```python
from build123d import *

# Parameters (mm, degrees)
SKETCH1_W           = 100
SKETCH1_H           = 80
BOSS_EXTRUDE1_DEPTH = 55
SKETCH3_W           = 90
SKETCH3_H           = 70
CUT_EXTRUDE1_DEPTH  = 50
SKETCH5_R           = 1.5
CUT_EXTRUDE2_DEPTH  = 50


with BuildPart() as part:
    # Sketch1 → Boss-Extrude1 (new body)
    with BuildSketch(Plane(origin=(0, 0, 0), x_dir=(1, 0, 0), z_dir=(0, 1, 0))):
        Rectangle(SKETCH1_W, SKETCH1_H)
    extrude(amount=BOSS_EXTRUDE1_DEPTH)

    # Sketch3 → Cut-Extrude1 (cut)
    with BuildSketch(Plane(origin=(0, 55, 0), x_dir=(1, 0, 0), z_dir=(0, 1, 0))):
        Rectangle(SKETCH3_W, SKETCH3_H)
    extrude(amount=-CUT_EXTRUDE1_DEPTH, mode=Mode.SUBTRACT)

    # Sketch5 → Cut-Extrude2 (cut)
    with BuildSketch(Plane(origin=(0, 5, 0), x_dir=(1, 0, 0), z_dir=(0, 1, 0))):
        with Locations(Location((-34.701504138, 23.983302554, 0), (0, 0, 270))):
            Circle(SKETCH5_R)
        with Locations(Location((34.701504138, 23.983302554, 0), (0, 0, 270))):
            Circle(SKETCH5_R)
        with Locations(Location((34.701504138, -23.983302554, 0), (0, 0, 270))):
            Circle(SKETCH5_R)
        with Locations(Location((-34.701504138, -23.983302554, 0), (0, 0, 270))):
            Circle(SKETCH5_R)
    extrude(amount=-CUT_EXTRUDE2_DEPTH, mode=Mode.SUBTRACT)


solid = part.part
```
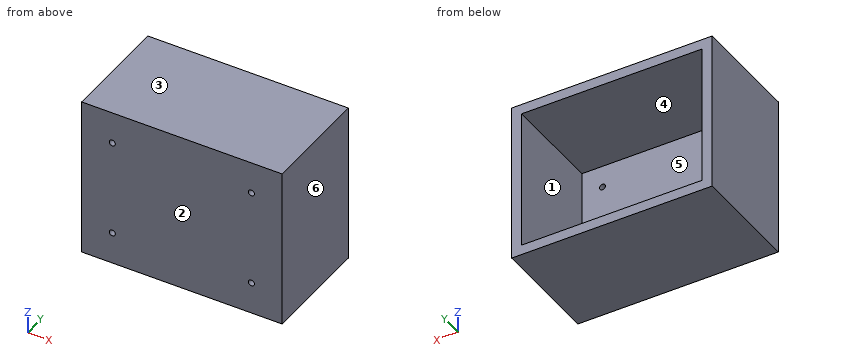
CAD build for the part. Positions are in the model's coordinates, mm. Face numbers are marked on the shaded views. A direction names the side the tool comes from. Coordinates: 2 decimals unless noted, no trailing zeros. Write each loop counter-clockwise with the first axis right and the second up, starting at its lowest first coordinate (ties: lowest second). Pieces come first, ordered by that corner, then holes. Notation, with made-up numbers: (-11.75, 80.5) -> (40.25, 80.5) arc R20 cw to (40.25, 94.5) -> close; hole circle Ø2 at (70.5, 33). An arc over 180 degrees is marked (long way). Use CSV: the item, a comma, the result in double quotes. Start each with the question number.
Item 1: Band-saw the part on A-A, the plane y = 32. Write the cut outline in (x, z), plus the area to 3 significant figures.
Item 2: Tool access for the marked faces 5 and 6: list every direction of +Z, -Z, +X, -X, +Y, -Y with a clear straight run to the whole face (end or side of a thin tool).
Item 3: Band-saw the part on C-C, the plane x = 22.5. Write the cut outline in (y, z), plus the area to 3 significant figures.
Item 4: Two-plate mould, pull along Z, no slides. Class the marked faces 1, 2, 3 and 4: +Z half, -Z half, draft (parallel to the pull), parting line (faces both ways), or undercut.
Item 5: Band-saw the part on B-B, the plane z = 4.5. Write the cut outline in (x, y), plus the area to 3 significant figures.
Item 6: Wall check: probe 1 along X at (y, z) = (48.5, 1); probe 2 along Z at (x, y) = (32, 27.5); probe 3 along X at (y, z) = (2.5, -24.5). Give the ranges that are in metal, low to high.
Item 7: Drop a flat-ended pin along its axis: P1, Ø1, axis at x = -28, z = -1, coming from the +Y side. Give the stop position or say it passes through.
Response values:
1,outline,"(-50, -40) -> (50, -40) -> (50, 40) -> (-50, 40) -> close; hole (-45, -35) -> (45, -35) -> (45, 35) -> (-45, 35) -> close"
1,area,"1,700 mm2"
2,face 5,"+Y"
2,face 6,"+Z, -Z, +X, +Y, -Y"
3,outline,"(0, -40) -> (55, -40) -> (55, -35) -> (5, -35) -> (5, 35) -> (55, 35) -> (55, 40) -> (0, 40) -> close"
3,area,"900 mm2"
4,face 1,"undercut"
4,face 2,"draft"
4,face 3,"+Z half"
4,face 4,"undercut"
5,outline,"(-50, 0) -> (50, 0) -> (50, 55) -> (45, 55) -> (45, 5) -> (-45, 5) -> (-45, 55) -> (-50, 55) -> close"
5,area,"1,000 mm2"
6,probe 1,"x = -50 to -45, 45 to 50"
6,probe 2,"z = -40 to -35, 35 to 40"
6,probe 3,"x = -50 to -36.11, -33.29 to 33.29, 36.11 to 50"
7,P1,"stops at y = 5"
